Can you work these out from the drawing? Everything is in mm from the part's minimum corner. Round coordinates to 2 decimals unless told otherwise and drop trailing zeros. Write each loop counter-clockwise with the first axis right and the second up, starting at its lowest first coordinate (ties: lowest second). Pieces come first, ordered by that corner, then holes. Notation, with made-up numbers: (-20.75, 0) - (22.25, 0) arc R7 cw to (22.25, 7) - close; hole circle Ø10 at (44.25, 32.25). An arc over 180 degrees is marked (long way). One line per item, written item: value. Start each with the question number.
(1) I want a section at A-A on y = 15. List the corners of the cut face in (x, z) for me.
(2) Thinking about a two-plate mould opening in X: for the marked faces 1, 2, 3 and 4, which applies, +X half, -X half, draft (parallel to the pull), parting line (faces both ways), or undercut?
(3) If I drill on L1, parallel to Z at x = 173.5, y = 111; L2, parallel to Y at x = 139, z = 87; L3, parallel to Y at x = 112, z = 18, over which ranges is the centre line in solid material (lowest first)? Write a range as from..to.
(4) I want a section at D-D on y = 57. List the corners of the cut face in (x, z) for me, plus the area to 3 significant figures.
(5) I want a section at C-C on x = 155. List the corners of the cut face in (y, z) for me, plus the area to 3 significant figures.
(6) I want a section at B-B on z = 59.5. List the corners of the cut face in (x, y) for me.
(7) I'm going to push flat-ended pins straight in: pin 1 Ø15 at (y, z) = (9.5, 70) entering from -X; pin 2 Ø15 at (x, z) = (82, 101) entering from -Y; pin 3 Ø24 at (x, z) = (162, 99.5) entering from +Y. Where does each tip first touch, or does it pass through?
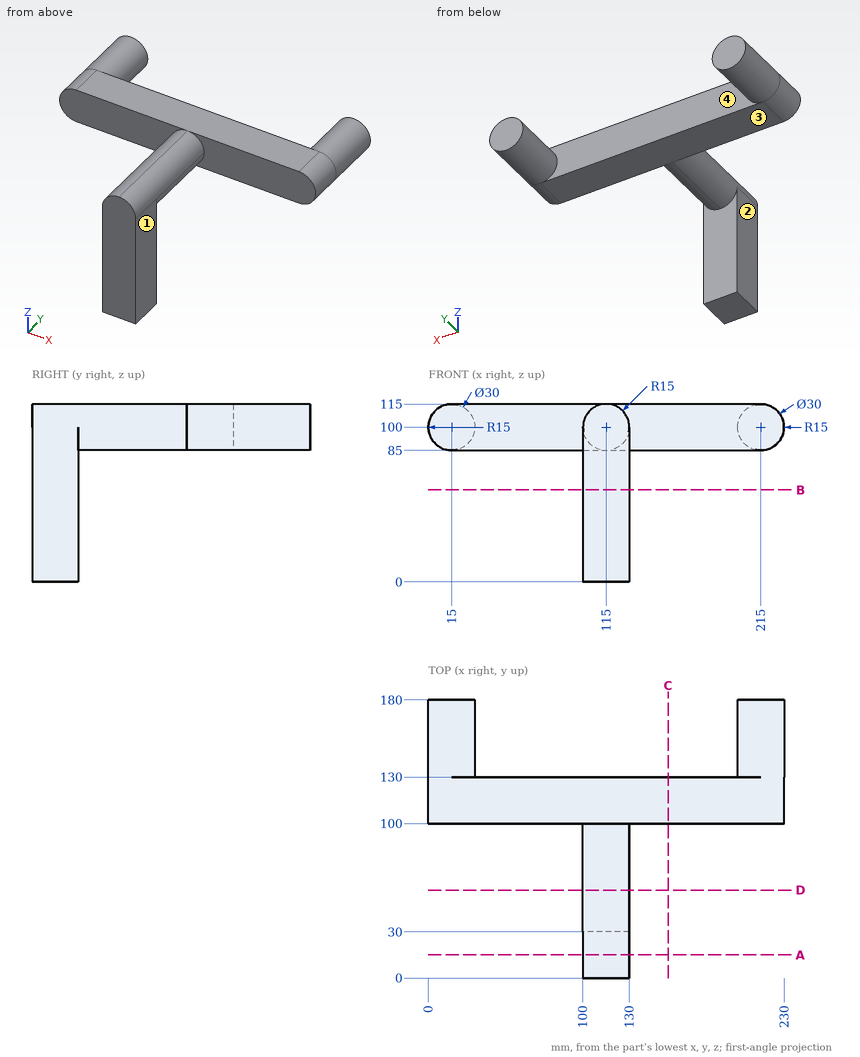
Established:
1. outline: (100, 0) - (130, 0) - (130, 100) arc R15 ccw to (100, 100) - close
2. face 1: +X half
2. face 2: -X half
2. face 3: draft
2. face 4: undercut
3. L1: 85..115
3. L2: 100..130
3. L3: 0..30
4. outline: (115, 115) arc R15 ccw (long way) to (130, 100) arc R15 ccw to start
4. area: 707 mm2
5. outline: (100, 85) - (130, 85) - (130, 115) - (100, 115) - close
5. area: 900 mm2
6. outline: (100, 0) - (130, 0) - (130, 30) - (100, 30) - close
7. pin 1: x = 100
7. pin 2: y = 100
7. pin 3: y = 130
